Build history of the part. All positions in model axes, mm. Give positions to 0.01 mm unless a question says otherwise; leave off trailing zeros. Loops run counter-clockwise (first coordinate to the right, second up) from the corner with the lowest first, then second, coordinate; pieces in that order, holes last.
1) Band-saw the part on C-C on z = 0.95. List the corners of the cut face in (x, y), then the cut area to 3 significant figures.
2) Wall check: line 1 (X direction, y = 45.5, z = 0.85); line 2 (Y direction, x = -6.5, z = 0.7); line 3 (X direction, y = 67, z = 0.7). Give the ranges that are in metal, low to high.
3) Band-saw the part on B-B on x = -6. List the corners of the cut face in (y, z).
4) Band-saw the part on A-A on y = 37. List the corners of the cut face in (x, z).
5) Flat gauge pins, fed straight in: P1, Ø2.5, axis at x = -73.22, y = 83.31, coming from the +Z side; P2, Ø4, axis at x = -52.22, y = 32.41, coming from the +Z side. Where does each tip first touch, or does it go through?
```python
from build123d import *

# Parameters (mm, degrees)
SKETCH1_W                                         = 100
SKETCH1_H                                         = 90
BOSS_EXTRUDE1_DEPTH                               = 2
SKETCH2_R                                         = 25.4
CUT_EXTRUDE1_DEPTH                                = 3
SKETCH3_R                                         = 1.5
CUT_EXTRUDE2_DEPTH                                = 3
SKETCH4_R                                         = 1.5
CUT_EXTRUDE3_DEPTH                                = 10
CSK_FOR_0_FLAT_HEAD_MACHINE_SCREW_100_D           = 1.778
CSK_FOR_0_FLAT_HEAD_MACHINE_SCREW_100_CSINK_D     = 3.0226
CSK_FOR_0_FLAT_HEAD_MACHINE_SCREW_100_CSINK_ANGLE = 100


with BuildPart() as part:
    # Sketch1 → Boss-Extrude1 (new body)
    with BuildSketch(Plane.XY):
        with Locations((-26.224709151, 41.314420924)):
            Rectangle(SKETCH1_W, SKETCH1_H)
    extrude(amount=BOSS_EXTRUDE1_DEPTH)

    # Sketch2 → Cut-Extrude1 (cut)
    with BuildSketch(Plane.XY.offset(2)):
        with Locations((-26.224709151, 46.314420924)):
            Circle(SKETCH2_R)
    extrude(amount=-CUT_EXTRUDE1_DEPTH, mode=Mode.SUBTRACT)

    # Sketch3 → Cut-Extrude2 (cut)
    with BuildSketch(Plane.XY.offset(2)):
        with Locations((-52.224709151, 32.414420924)):
            Circle(SKETCH3_R)
        with Locations((-0.224709151, 32.414420924)):
            Circle(SKETCH3_R)
    extrude(amount=-CUT_EXTRUDE2_DEPTH, mode=Mode.SUBTRACT)

    # Sketch4 → Cut-Extrude3 (cut)
    with BuildSketch(Plane(origin=(0, 0, 0), x_dir=(-1, 0, 0), z_dir=(0, 0, -1))):
        with Locations((-20.775290849, 83.314420924)):
            Circle(SKETCH4_R)
        with Locations((73.224709151, 83.314420924)):
            Circle(SKETCH4_R)
        with Locations((73.224709151, -0.685579076)):
            Circle(SKETCH4_R)
        with Locations((-20.775290849, -0.685579076)):
            Circle(SKETCH4_R)
    extrude(amount=-CUT_EXTRUDE3_DEPTH, mode=Mode.SUBTRACT)

    # CSK for #0 Flat Head Machine Screw (100)2 (through all)
    with Locations(Plane(origin=(0, 0, 0), x_dir=(-1, 0, 0), z_dir=(0, 0, -1))):
        with Locations((-20.775290849, 83.314420924), (73.224709151, 83.314420924), (73.224709151, -0.685579076), (-20.775290849, -0.685579076)):
            CounterSinkHole(CSK_FOR_0_FLAT_HEAD_MACHINE_SCREW_100_D / 2, CSK_FOR_0_FLAT_HEAD_MACHINE_SCREW_100_CSINK_D / 2, counter_sink_angle=CSK_FOR_0_FLAT_HEAD_MACHINE_SCREW_100_CSINK_ANGLE)


solid = part.part
```
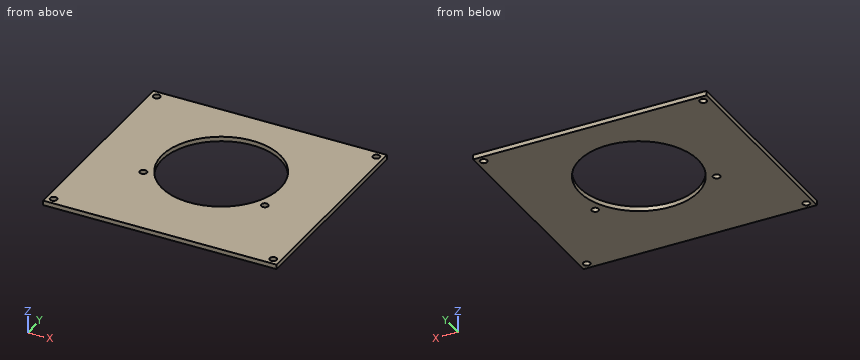
Findings below:
1. outline: (-76.22, -3.69) - (23.78, -3.69) - (23.78, 86.31) - (-76.22, 86.31) - close; hole circle Ø3 at (-73.22, -0.69); hole circle Ø3 at (-73.22, 83.31); hole circle Ø3 at (-52.22, 32.41); hole circle Ø50.8 at (-26.22, 46.31); hole circle Ø3 at (-0.22, 32.41); hole circle Ø3 at (20.78, -0.69); hole circle Ø3 at (20.78, 83.31)
1. area: 6,930 mm2
2. line 1: x = -76.22 to -51.61, -0.84 to 23.78
2. line 2: y = -3.69 to 30.31, 62.32 to 86.31
2. line 3: x = -76.22 to -40.96, -11.48 to 23.78
3. outline: (-3.69, 0) - (30.95, 0) - (30.95, 2) - (-3.69, 2) - close; (61.68, 0) - (86.31, 0) - (86.31, 2) - (61.68, 2) - close
4. outline: (-76.22, 0) - (-49.86, 0) - (-49.86, 2) - (-76.22, 2) - close; (-2.59, 0) - (23.78, 0) - (23.78, 2) - (-2.59, 2) - close
5. P1: passes through
5. P2: stops at z = 2
